Build history of the part. All positions in model axes, mm. A direction names the side the tool comes from. Give positions to 0.01 mm unless a question says otherwise; leave off trailing zeros. Order: outer loops, then holes, each group sorted by start corner. A loop starts at its lowest first (then second) coordinate and runs counter-clockwise, first axis right, second up. Notation, with made-up numbers: (37, 73) -> (52, 73) arc R24 cw to (52, 97) -> close; hole circle Ø8 at (-4.5, 77). An arc over 180 degrees is marked (long way). One line per item, written item: value. Start each with the question number.
(1) Saw through at C-C on x = 34.5. Give the cut face in (y, z), plus the area to 3 significant figures.
(2) Saw through at A-A on x = 16.5. Give the cut face in (y, z), plus the area to 3 significant figures.
(3) Two-plate mould, pull along Z, no slides. Class faces 1 (the flat face through (25, -54, 0)), 2 (the flat face through (37, -48, -49)), 3 (the flat face through (17, -58, -90.989)): +Z half, -Z half, draft (parallel to the pull), parting line (faces both ways), or undercut.
(4) Probe line 1 (Z direction, x = 15.5, y = -59); line 2 (Y direction, x = 14.5, z = -94.5); line 3 (Y direction, x = 31.5, z = -13). List the from-to ranges inside material, lowest first.
(5) Saw through at B-B on y = -49.75. Give the cut face in (x, z).
(6) Pin check, flat tips, straight feed: pin 1 (10 mm diameter, centred on x = 33.5, z = -47, fed in from -Y); pin 2 (8 mm diameter, centred on y = -52, z = -87, fed in from +X); pin 3 (1.5 mm diameter, centred on x = 25, z = -82, fed in from -Y). Stop position of each tip, or through.
(7) Which spindle directions (+Z, -Z, +X, -X, +Y, -Y) get a long thin tool onto all of the face, cutting with end or side? Do faces 4 (the cylindrical face through (26.501, -53.116, -98.158)), 5 (the flat face through (21.66, -55.7, -75.8)). Say none if no direction does.
Autodesk Inventor part; units mm, degrees
ref_plane "YZ Plane" through (0, 0, 0) normal (1, 0, 0) x (0, 1, 0)
ref_plane "XZ Plane" through (0, 0, 0) normal (0, 1, 0) x (-1, 0, 0)
ref_plane "XY Plane" through (0, 0, 0) normal (0, 0, 1) x (1, 0, 0)
sketch "Szkic1" plane through (0, 0, 0) normal (0, 0, 1) x (1, 0, 0)
  line L0 (0, 0) -> (0, -66.5)
  line L1 (0, -66.5) -> (2, -66.5)
  line L2 (2, 0) -> (2, -66.5)
  line L3 (0, 0) -> (2, 0)
  circle A0 centre (7, 15.8) radius 1.5
  circle A1 centre (7, 15.8) radius 15.02
  line L4 (7, 30.82) -> (7, 14.3)
  line L5 (7, -69.18) -> (-7.0129, -69.18)
  line L6 (37, -46.3508) -> (4.3309, -63.8229)
  line L7 (37, -48.6189) -> (3.5105, -66.5297)
  line L8 (37, -48.6189) -> (37, -46.3508)
  line L9 (37, -48.6189) -> (-1.4451, -69.18)
  line L10 (37, -46.3508) -> (-1.4451, -66.9119)
  line L11 (-1.4451, -66.9119) -> (-1.4451, -69.18)
  dimension "d0" = 100
extrude "Wyciągnięcie proste1" add sketch "Szkic1" against normal blind 100 contours L10 L2 L1 L0 | L0 L1 L2 L10 L6 L8 L7 L9 L11
sketch "Szkic5" plane through (-1.4451, -69.18, -100) normal (0.4716076, -0.8818085, 0) x (0.8818085, 0.4716076, 0)
  line L0 (17.9345, 9.0111) -> (17.7164, 38.6148)
  line L1 (17.7164, 38.6148) -> (26.2335, 38.9662)
  line L2 (26.4517, 9.3625) -> (17.9345, 9.0111)
  line L3 (26.2335, 38.9662) -> (17.9345, 38.9662)
  line L4 (17.9345, 38.9662) -> (17.9345, 9.0111)
  line L5 (17.9345, 9.0111) -> (26.2335, 9.0111)
  line L6 (26.2335, 9.0111) -> (26.2335, 38.9662)
  line L7 (17.4345, 39.4662) -> (26.7335, 39.4662)
  line L8 (26.7335, 39.4662) -> (26.7335, 8.5111)
  line L9 (26.7335, 8.5111) -> (17.4345, 8.5111)
  line L10 (17.4345, 8.5111) -> (17.4345, 39.4662)
  line L11 (17.4345, 39.4662) -> (16.9345, 39.4662)
  line L12 (16.9345, 39.4662) -> (16.9345, 8.5111)
  line L13 (16.9345, 8.5111) -> (17.4345, 8.5111)
  line L14 (17.4345, 8.5111) -> (17.4345, 39.4662)
  line L15 (26.7335, 38.9662) -> (16.9345, 38.9662)
  line L16 (16.9345, 38.9662) -> (16.9345, 9.0111)
  line L17 (16.9345, 9.0111) -> (26.7335, 9.0111)
  line L18 (26.7335, 9.0111) -> (26.7335, 38.9662)
  point P0 (33.9001, 100)
  point P1 (17.9345, 9.0111)
  point P2 (26.7335, 9.0111)
  point P3 (17.9345, 38.9662)
  dimension "d7" = 0.5
  dimension "d8" = 0.5
extrude "Wyciągnięcie proste4" cut sketch "Szkic5" against normal through all contours L17 L10 L15 L4 L1 L0 | L4 L1 L6 L2 | L0 L1 L4 | L2 L6 L5 | L6 L15 L8 L17 | L4 L3 L1 | L17 L12 L15 L10
ref_plane "Płaszczyzna konstrukcyjna1" through (0, 0, -50) normal (0, 0, 1) x (1, 0, 0)
mirror "Odbij1" about plane through (0, 0, -50) normal (0, 0, 1) of "Wyciągnięcie proste4"
sketch "Szkic6" plane through (-1.4451, -69.18, -100) normal (0.4716076, -0.8818085, 0) x (0.8818085, 0.4716076, 0)
  line L0 (0, 100) -> (1.0696, 100)
  line L1 (0, 100) -> (0, 0)
  line L2 (1.0696, 0) -> (0, 0)
  line L3 (1.0696, 0) -> (44.6676, 0)
  line L4 (0, 100) -> (16.9345, 100)
  line L5 (16.9345, 100) -> (16.9345, 0)
  line L6 (16.9345, 0) -> (0, 0)
  line L7 (0, 0) -> (0, 100)
  line L8 (0, 0) -> (1.0696, 0)
  line L9 (0, 0) -> (-9.525, 0)
  line L10 (-9.525, 0) -> (-9.525, 100)
  line L11 (-9.525, 100) -> (0, 100)
  line L12 (0, 100) -> (0, 0)
  line L13 (1.0696, 0) -> (1.0696, 100)
  point P0 (33.9001, 100)
  point P1 (43.598, 0)
  point P2 (16.9345, 0)
  point P3 (0, 100)
  point P4 (16.9345, 61.0338)
  point P5 (16.9345, 90.9889)
  point P6 (16.9345, 9.0111)
  point P7 (16.9345, 38.9662)
extrude "Wyciągnięcie proste5" cut sketch "Szkic6" against normal through all
sketch "Szkic7" plane through (37, -48.6189, -100) normal (0.4716076, -0.8818085, 0) x (0.8818085, 0.4716076, 0)
  line L0 (-26.6634, 90.9889) -> (-16.8645, 90.9889)
  line L1 (-16.8645, 90.9889) -> (-16.8645, 61.0338)
  line L2 (-16.8645, 61.0338) -> (-26.6634, 61.0338)
  line L3 (-26.6634, 38.9662) -> (-16.8645, 38.9662)
  line L4 (-16.8645, 38.9662) -> (-16.8645, 9.0111)
  line L5 (-16.8645, 9.0111) -> (-26.6634, 9.0111)
  line L6 (0, 0) -> (-26.6634, 0)
  line L7 (0, 100) -> (0, 0)
  line L8 (-26.6634, 100) -> (0, 100)
  line L9 (-26.6634, 90.9889) -> (-26.6634, 100)
  line L10 (0, 100) -> (-26.6634, 100)
  line L11 (-26.6634, 100) -> (-26.6634, 92.9)
  line L12 (-26.6634, 92.9) -> (0, 92.9)
  line L13 (0, 92.9) -> (0, 100)
  line L14 (-16.8645, 90.9889) -> (-16.8645, 100)
  line L15 (1.0696, 100) -> (-42.5283, 100)
  circle A0 centre (-11, 96.45) radius 1.75
  line L16 (-52.6978, 50) -> (11.0012, 50)
  circle A1 centre (-11, 3.55) radius 1.75
  line L17 (-26.6634, 100) -> (-26.6634, 90.9889)
  line L18 (-26.6634, 61.0338) -> (-26.6634, 38.9662)
  line L19 (-26.6634, 9.0111) -> (-26.6634, 0)
  point P0 (-9.6979, 100)
  point P1 (0, 96.45)
  dimension "d13" = 7.1
  dimension "d15" = 11
  dimension "d16" = 3.55
  dimension "d17" = 3.5
extrude "Wyciągnięcie proste6" cut sketch "Szkic7" against normal through all contours A0 | A1
sketch "Szkic8" plane through (37, -46.3508, 0) normal (-0.4716076, 0.8818085, 0) x (0.8818085, 0.4716076, 0)
  circle A0 centre (-12.0696, 96.45) radius 1.75
  circle A1 centre (-12.0696, 3.55) radius 1.75
  line L0 (-27.7331, 9.0111) -> (-27.7331, 0)
  line L1 (0, 0) -> (-27.7331, 0)
  line L2 (0, 0) -> (0, 100)
  line L3 (-27.7331, 100) -> (0, 100)
  line L4 (-27.7331, 100) -> (-27.7331, 90.9889)
  line L5 (-27.7331, 90.9889) -> (-17.9341, 90.9889)
  line L6 (-17.9341, 90.9889) -> (-17.9341, 61.0338)
  line L7 (-17.9341, 61.0338) -> (-27.7331, 61.0338)
  line L8 (-27.7331, 61.0338) -> (-27.7331, 38.9662)
  line L9 (-27.7331, 38.9662) -> (-17.9341, 38.9662)
  line L10 (-17.9341, 38.9662) -> (-17.9341, 9.0111)
  line L11 (-17.9341, 9.0111) -> (-27.7331, 9.0111)
  point P0 (-10.7675, 0)
properties part number "plug_2"
Results below:
1. outline: (-49.96, -100) -> (-47.69, -100) -> (-47.69, 0) -> (-49.96, 0) -> close
1. area: 227 mm²
2. outline: (-59.58, -100) -> (-57.31, -100) -> (-57.31, -90.99) -> (-59.58, -90.99) -> close; (-59.58, -61.03) -> (-57.31, -61.03) -> (-57.31, -38.97) -> (-59.58, -38.97) -> close; (-59.58, -9.01) -> (-57.31, -9.01) -> (-57.31, 0) -> (-59.58, 0) -> close
2. area: 90.9 mm²
3. face 1: +Z half
3. face 2: draft
3. face 3: undercut
4. line 1: z = -100 to -90.99, -61.03 to -38.97, -9.01 to 0
4. line 2: y = -60.65 to -58.38
4. line 3: y = -51.56 to -49.29
5. outline: (30.64, -100) -> (34.89, -100) -> (34.89, 0) -> (30.64, 0) -> close
6. pin 1: stops at y = -53.16
6. pin 2: stops at x = 37
6. pin 3: stops at y = -55.44
7. face 4: none
7. face 5: -X, -Y
